Source: CAD feature listing. Evaluate the final solid. Frame: model axes, mm. Face numbers are marked on the shaded views. A direction names the side the tool comes from. Give positions to 0.01 mm unless a question says otherwise; leave off trailing zeros. Order: outer loops, then holes, each group sorted by start corner. A loop starts at its lowest first (then second) coordinate and runs counter-clockwise, first axis right, second up.
1) Section A-A, the plane y = 41.91. Return loops of the section in (x, z) (3 decimals).
2) Section D-D, the plane y = 34.5. Return loops of the section in (x, z) (3 decimals).
3) Section C-C, the plane z = -8.89. Return loops of the section in (x, y) (3 decimals).
4) Access query for the marked faces 1, 2, 3 and 4. Directions: +Z, -Z, +X, -X, +Y, -Y. A direction counts if a zero-diameter tool reaches every point of the face in a straight line with its end or side. Return the directions, or none.
5) Material intervals for line 1 (Z direction, x = 41.91, y = -2.1); line 2 (Y direction, x = -1.1, z = -8.89); line 3 (Y direction, x = -2, z = -8), sorted ascending.
6) First-contact query: P1, Ø6, axis at x = 23.5, y = 6.5, coming from the -Z side; P2, Ø14, axis at x = 39, z = -11, coming from the +Y side; P3, Ø5, axis at x = 10.5, y = 19.5, coming from the +Z side. Flat tips, straight axial feed; report the tip coordinate or a pass-through.
```python
from build123d import *

# Parameters (mm, degrees)
BOSS_EXTRUDE1_DEPTH = 6.35
SKETCH2_W           = 41.91
SKETCH2_H           = 17.78
BOSS_EXTRUDE2_DEPTH = 3.175
SKETCH3_W           = 17.78
SKETCH3_H           = 41.91
BOSS_EXTRUDE3_DEPTH = 3.175
SKETCH4_R           = 3.3782
CUT_EXTRUDE1_DEPTH  = 3.175
SKETCH5_R           = 3.3782
CUT_EXTRUDE2_DEPTH  = 3.175


with BuildPart() as part:
    # Sketch1 → Boss-Extrude1 (new body)
    with BuildSketch(Plane.XY):
        with BuildLine():
            Line((0, 5.08), (0, 50.8))
            Line((0, 50.8), (50.8, 0))
            Line((50.8, 0), (5.08, 0))
            ThreePointArc((5.08, 0), (1.487897552, 1.487897552), (0, 5.08))
        make_face()
    extrude(amount=BOSS_EXTRUDE1_DEPTH)

    # Sketch2 → Boss-Extrude2 (add)
    with BuildSketch(Plane.ZY):
        with Locations((3.175, 41.91)):
            Rectangle(SKETCH2_W, SKETCH2_H)
    extrude(amount=BOSS_EXTRUDE2_DEPTH)

    # Sketch3 → Boss-Extrude3 (add)
    with BuildSketch(Plane.XZ):
        with Locations((41.91, 3.175)):
            Rectangle(SKETCH3_W, SKETCH3_H)
    extrude(amount=BOSS_EXTRUDE3_DEPTH)

    # Sketch4 → Cut-Extrude1 (cut)
    with BuildSketch(Plane(origin=(0, 0, 0), x_dir=(1, 0, 0), z_dir=(0, 1, 0))):
        with Locations((41.91, 8.89)):
            Circle(SKETCH4_R)
        with Locations((41.91, -15.24)):
            Circle(SKETCH4_R)
    extrude(amount=-CUT_EXTRUDE1_DEPTH, mode=Mode.SUBTRACT)

    # Sketch5 → Cut-Extrude2 (cut)
    with BuildSketch(Plane(origin=(0, 0, 0), x_dir=(0, 0, -1), z_dir=(1, 0, 0))):
        with Locations((-15.24, 41.91)):
            Circle(SKETCH5_R)
        with Locations((8.89, 41.91)):
            Circle(SKETCH5_R)
    extrude(amount=-CUT_EXTRUDE2_DEPTH, mode=Mode.SUBTRACT)


solid = part.part
```
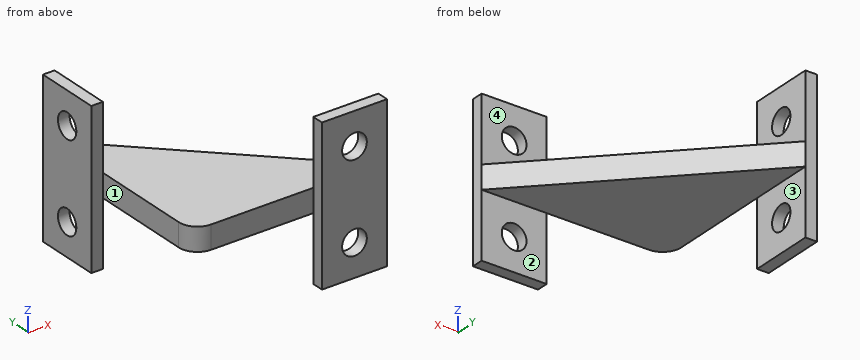
From the geometry:
1. outline: (-3.175, -17.78) - (0, -17.78) - (0, -12.268) - (-3.175, -12.268) - close; (-3.175, -5.512) - (0, -5.512) - (0, 0) - (8.89, 0) - (8.89, 6.35) - (0, 6.35) - (0, 11.862) - (-3.175, 11.862) - close; (-3.175, 18.618) - (0, 18.618) - (0, 24.13) - (-3.175, 24.13) - close
2. outline: (-3.175, -17.78) - (0, -17.78) - (0, 0) - (16.3, 0) - (16.3, 6.35) - (0, 6.35) - (0, 24.13) - (-3.175, 24.13) - close
3. outline: (-3.175, 33.02) - (0, 33.02) - (0, 38.532) - (-3.175, 38.532) - close; (-3.175, 45.288) - (0, 45.288) - (0, 50.8) - (-3.175, 50.8) - close; (33.02, -3.175) - (38.532, -3.175) - (38.532, 0) - (33.02, 0) - close; (45.288, -3.175) - (50.8, -3.175) - (50.8, 0) - (45.288, 0) - close
4. face 1: +Z, -Z, -X, -Y
4. face 2: -Z, +X, -X, +Y
4. face 3: -Z, +X, +Y, -Y
4. face 4: +Z, +X, -X, +Y
5. line 1: z = -17.78 to -12.27, -5.51 to 11.86, 18.62 to 24.13
5. line 2: y = 33.02 to 38.53, 45.29 to 50.8
5. line 3: y = 33.02 to 38.65, 45.17 to 50.8
6. P1: stops at z = 0
6. P2: stops at y = 0
6. P3: stops at z = 6.35
